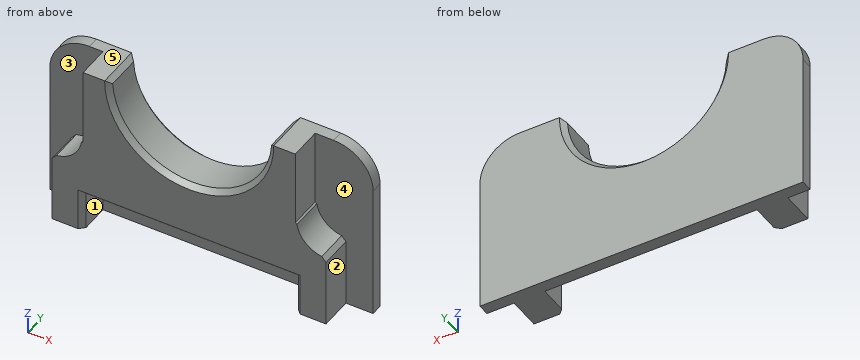
```python
from build123d import *

# Parameters (mm, degrees)
F0_W         = 124.8875334859
F0_H         = 67.7581354976
F1_DEPTH     = 4.445
F2_R         = 15.24
F4_DEPTH     = 12.7
F6_DEPTH     = 50.8
F8_DEPTH     = 12.7
F9_T1_DEPTH  = 26.6729642247
F9_T3_DEPTH  = 19.5947973283
F9_T5_DEPTH  = 81.9930359721
F9_T7_DEPTH  = 17.2644261819
F9_T10_ANGLE = 198.2651986278
F9_T12_ANGLE = 198.2651986278
F9_T16_DEPTH = 17.2644261819
F9_T21_DEPTH = 17.2644261819
F9_T27_DEPTH = 86.8920920642
F9_T31_DEPTH = 19.5947973283
F9_T38_DEPTH = 19.5947973283
F9_T42_DEPTH = 86.8920920642


# Not quite as in the source:
# - a fillet or chamfer that OpenCascade refuses, or shapes differently, is made with other operations: its cross-section is extruded or revolved along the edge and cut away or added


with BuildPart() as f1:
    # F0 (on Front) → F1 (new body)
    with BuildSketch(Plane.XZ):
        with Locations((0.9489916265, 33.8790677488)):
            Rectangle(F0_W, F0_H)
    extrude(amount=F1_DEPTH)

    # F2
    f2_edges = [f1.edges().sort_by_distance(p)[0] for p in [
        (-61.494775, -2.2225, 67.758135),
        (63.392758, -2.2225, 67.758135),
    ]]
    fillet(f2_edges, radius=F2_R)

    # F3 (on face) → F4 (join)
    with BuildSketch(Plane.XZ.offset(4.445)):
        Polygon((40.9965217113, 67.7581354976), (-40.9965142608, 67.7581354976), (-40.9965142608, 39.0565320849), (-40.9965142608, 14.6957412362), (40.9965217113, 14.6957412362), (40.9965217113, 39.4814237952), align=None)
        Polygon((-40.9965142608, 14.6957412362), (-40.9965142608, 39.0565320849), (-52.9372058809, 39.0565320849), (-52.9372058809, 0), (-40.9965142608, 0), align=None)
        Polygon((52.8750233352, 39.4814237952), (40.9965217113, 39.4814237952), (40.9965217113, 14.6957412362), (40.9965217113, 0), (52.8750233352, 0), align=None)
    extrude(amount=F4_DEPTH)

    # F5 (on face) → F6 (cut)
    with BuildSketch(Plane.XZ.offset(17.145)):
        with BuildLine():
            ThreePointArc((-30.7849538809, 67.7581354976), (0, 36.9731816167), (30.7849538809, 67.7581354976))
            Line((30.7849538809, 67.7581354976), (-30.7849538809, 67.7581354976))
        make_face()
        with BuildLine():
            Line((-30.7849538809, 67.7581354976), (30.7849538809, 67.7581354976))
            ThreePointArc((30.7849538809, 67.7581354976), (0, 98.5430893784), (-30.7849538809, 67.7581354976))
        make_face()
    extrude(amount=-F6_DEPTH, mode=Mode.SUBTRACT)

    # F7 (on face) → F8 (cut)
    with BuildSketch(Plane.XZ.offset(17.145)):
        with BuildLine():
            ThreePointArc((-52.9372058809, 27.6993892785), (-44.9064931875, 31.0258193916), (-41.5800630744, 39.0565320849))
            Line((-41.5800630744, 39.0565320849), (-52.9372058809, 39.0565320849))
            Line((-52.9372058809, 39.0565320849), (-52.9372058809, 27.6993892785))
        make_face()
        with BuildLine():
            Line((52.8750233352, 39.4814237952), (41.5178805288, 39.4814237952))
            ThreePointArc((41.5178805288, 39.4814237952), (44.8443106419, 31.4507111019), (52.8750233352, 28.1242809888))
            Line((52.8750233352, 28.1242809888), (52.8750233352, 39.4814237952))
        make_face()
    extrude(amount=-F8_DEPTH, mode=Mode.SUBTRACT)

    # F9: chamfer of 1.905 on 11 edges, made by hand

    # F9_s2 → F9_t1 (cut)
    with BuildSketch(Plane.XZ.offset(-4.7639821123)):
        with BuildLine():
            Line((-32.6343999444, 67.7581354976), (-30.7326373381, 65.964148961))
            ThreePointArc((-30.7326373381, 65.964148961), (-30.7710738122, 66.8337968736), (-30.7849538809, 67.7581354976))
            Line((-30.7849538809, 67.7581354976), (-32.6343999444, 67.7581354976))
        make_face()
        with BuildLine():
            Line((30.7326373381, 65.964148961), (32.6343999444, 67.7581354976))
            Line((32.6343999444, 67.7581354976), (30.7849538809, 67.7581354976))
            ThreePointArc((30.7849538809, 67.7581354976), (30.7710738122, 66.8337968736), (30.7326373381, 65.964148961))
        make_face()
    extrude(amount=F9_T1_DEPTH, mode=Mode.SUBTRACT)

    # F9_s4 → F9_t3 (cut)
    with BuildSketch(Plane.XY.offset(-4.8990560921)):
        Polygon((-42.9015142608, -17.145), (-40.9965142608, -15.24), (-40.9965142608, -17.145), align=None)
        Polygon((42.9015217113, -17.145), (40.9965217113, -15.24), (40.9965217113, -17.145), align=None)
    extrude(amount=F9_T3_DEPTH, mode=Mode.SUBTRACT)

    # F9_s6 → F9_t5 (cut)
    with BuildSketch(Plane.YZ.offset(-40.9965142608)):
        Polygon((-17.145, 16.6007412362), (-15.24, 14.6957412362), (-17.145, 14.6957412362), align=None)
    extrude(amount=F9_T5_DEPTH, mode=Mode.SUBTRACT)

    # F9_s8 → F9_t7 (cut)
    with BuildSketch(Plane.XZ.offset(4.445)):
        with BuildLine():
            Line((52.8750233352, 26.356813065), (51.2436612422, 28.24205769))
            ThreePointArc((51.2436612422, 28.24205769), (52.0302167258, 28.1557452496), (52.8750233352, 28.1242809888))
            Line((52.8750233352, 28.1242809888), (52.8750233352, 26.356813065))
        make_face()
        with BuildLine():
            Line((-52.9372058809, 25.9319213547), (-51.3058437879, 27.8171659797))
            ThreePointArc((-51.3058437879, 27.8171659797), (-52.0923992715, 27.7308535393), (-52.9372058809, 27.6993892785))
            Line((-52.9372058809, 27.6993892785), (-52.9372058809, 25.9319213547))
        make_face()
    extrude(amount=F9_T7_DEPTH, mode=Mode.SUBTRACT)

    # F9_s9 → F9_t10 (revolve, cut)
    with BuildSketch(Plane(origin=(10.6182323587, 0, 66.0511732612), x_dir=(0, 1, 0), z_dir=(0.1587198459, 0, 0.9873236605))):
        Polygon((-15.24, 41.539514704), (-17.145, 43.444514704), (-17.145, 41.539514704), align=None)
    revolve(axis=Axis((0, -17.145, 67.7581354976), (0, -1, 0)), revolution_arc=F9_T10_ANGLE, mode=Mode.SUBTRACT)

    # F9_s11 → F9_t12 (revolve, cut)
    with BuildSketch(Plane(origin=(10.6182323587, 0, 66.0511732612), x_dir=(0, 1, 0), z_dir=(0.1587198459, 0, 0.9873236605))):
        Polygon((0, 43.444514704), (-1.905, 41.539514704), (0, 41.539514704), align=None)
    revolve(axis=Axis((0, 0, 67.7581354976), (0, -1, 0)), revolution_arc=F9_T12_ANGLE, mode=Mode.SUBTRACT)


with BuildPart() as f9_tool14:
    # F9_s15 → F9_t16 (new body)
    with BuildSketch(Plane.XZ.offset(21.7094261819)):
        with BuildLine():
            Line((41.63565723, 37.8500617022), (39.750412605, 39.4814237952))
            Line((39.750412605, 39.4814237952), (41.5178805288, 39.4814237952))
            ThreePointArc((41.5178805288, 39.4814237952), (41.5493447896, 38.6366171858), (41.63565723, 37.8500617022))
        make_face()
    extrude(amount=-F9_T16_DEPTH)

    split(bisect_by=Plane.YZ.offset(40.9965217113), keep=Keep.TOP)


with BuildPart() as f1_1:
    add(f1.part)

    # F9_t13: cut F9_tool14
    add(f9_tool14.part, mode=Mode.SUBTRACT)


with BuildPart() as f9_tool19:
    # F9_s20 → F9_t21 (new body)
    with BuildSketch(Plane.XZ.offset(21.7094261819)):
        with BuildLine():
            Line((-39.8125951507, 39.0565320849), (-41.6978397756, 37.4251699919))
            ThreePointArc((-41.6978397756, 37.4251699919), (-41.6115273352, 38.2117254755), (-41.5800630744, 39.0565320849))
            Line((-41.5800630744, 39.0565320849), (-39.8125951507, 39.0565320849))
        make_face()
    extrude(amount=-F9_T21_DEPTH)

    split(bisect_by=Plane.YZ.offset(-40.9965142608), keep=Keep.BOTTOM)


with BuildPart() as f1_2:
    add(f1_1.part)

    # F9_t18: cut F9_tool19
    add(f9_tool19.part, mode=Mode.SUBTRACT)


with BuildPart() as f9_tool25:
    # F9_s26 → F9_t27 (new body)
    with BuildSketch(Plane.YZ.offset(-45.8955703528)):
        Polygon((-17.145, 16.6007412362), (-15.24, 14.6957412362), (-17.145, 14.6957412362), align=None)
    extrude(amount=F9_T27_DEPTH)

    split(bisect_by=Plane.YZ.offset(-40.9965142608), keep=Keep.BOTTOM)


with BuildPart() as f9_tool29:
    # F9_s30 → F9_t31 (new body)
    with BuildSketch(Plane.XY):
        Polygon((-42.9015142608, -17.145), (-40.9965142608, -15.24), (-40.9965142608, -17.145), align=None)
    extrude(amount=F9_T31_DEPTH)

    split(bisect_by=Plane.XY.offset(14.6957412362), keep=Keep.TOP)


with BuildPart() as f9_tool25_1:
    add(f9_tool25.part)

    # F9_t33: intersect F9_tool29
    add(f9_tool29.part, mode=Mode.INTERSECT)


with BuildPart() as f1_3:
    add(f1_2.part)

    # F9_t23: cut F9_tool25
    add(f9_tool25_1.part, mode=Mode.SUBTRACT)


with BuildPart() as f9_tool36:
    # F9_s37 → F9_t38 (new body)
    with BuildSketch(Plane.XY.offset(19.5947973283)):
        Polygon((42.9015217113, -17.145), (40.9965217113, -15.24), (40.9965217113, -17.145), align=None)
    extrude(amount=-F9_T38_DEPTH)

    split(bisect_by=Plane.XY.offset(14.6957412362), keep=Keep.TOP)


with BuildPart() as f9_tool40:
    # F9_s41 → F9_t42 (new body)
    with BuildSketch(Plane.YZ.offset(-40.9965142608)):
        Polygon((-17.145, 16.6007412362), (-15.24, 14.6957412362), (-17.145, 14.6957412362), align=None)
    extrude(amount=F9_T42_DEPTH)

    split(bisect_by=Plane.YZ.offset(40.9965217113), keep=Keep.TOP)


with BuildPart() as f9_tool36_1:
    add(f9_tool36.part)

    # F9_t44: intersect F9_tool40
    add(f9_tool40.part, mode=Mode.INTERSECT)


with BuildPart() as f1_4:
    add(f1_3.part)

    # F9_t34: cut F9_tool36
    add(f9_tool36_1.part, mode=Mode.SUBTRACT)


solid = f1_4.part
```
Build history of the part. All positions in model axes, mm. Face numbers are marked on the shaded views. A direction names the side the tool comes from. Round coordinates to 2 decimals unless told otherwise and drop trailing zeros. Write each loop counter-clockwise with the first axis right and the second up, starting at its lowest first coordinate (ties: lowest second). Pieces come first, ordered by that corner, then holes. Notation, with made-up numbers: (40, -24.75) - (57, -24.75) arc R21 ccw to (57, -5.75) - close; hole circle Ø2 at (-24, 15.25). An arc over 180 degrees is marked (long way). Write each question's results on one line, items separated by ' | '. Start each with the question number.
Item 1: Drop flat-ended pins along their axis: P1, Ø6, axis at x = -56, z = 47.5, coming from the -Y side (3 decimals); P2, Ø5.5, axis at x = 6.5, y = -10, coming from the -Z side; P3, Ø24.5, axis at x = 53.5, z = 31, coming from the -Y side (3 decimals); P4, Ø1.5, axis at y = -9, z = 30, coming from the +X side. Give the stop position or say it passes through.
Item 2: Saw through at C-C (y = -12.25). Write the cut outline in (x, z), and give its area (3 significant figures).
Item 3: Wall check: L1, parallel to X at y = -15, z = 3.5; L2, parallel to Y at x = -49, z = 51 (3 decimals); L3, parallel to X at y = -15.25, z = 21.5. Give the ranges that are in metal, low to high. Write a range as [from, to].
Item 4: Saw through at B-B (z = 20.5). Write the cut outline in (x, y) (3 decimals).
Item 5: Mould opens along X. For the marked faces 1, 2 and 3 say: pulls with the +X half, pulls with the -X half, needs draft (parallel to the pull), parting line crosses it, or undercut.
Item 6: Saw through at D-D (z = 13). Write the cut outline in (x, y) (3 decimals).
Item 7: Saw through at A-A (x = 0). Write the cut outline in (y, z) (3 decimals).
Item 8: Which spindle directions (+Z, -Z, +X, -X, +Y, -Y) get a long thin tool onto all of the face, cutting with end or side? Do the marked faces 4 and 5. Say none if no direction does.
Results are:
1) P1: stops at y = -4.445 | P2: stops at z = 14.7 | P3: stops at y = -17.145 | P4: stops at x = 47.95
2) outline: (-52.94, 0) - (-41, 0) - (-41, 14.7) - (41, 14.7) - (41, 0) - (52.88, 0) - (52.88, 26.36) - (51.24, 28.24) arc R11.36 cw to (41.64, 37.85) - (41, 38.4) - (41, 67.76) - (32.63, 67.76) - (30.73, 65.96) arc R30.78 cw to (-30.73, 65.96) - (-32.63, 67.76) - (-41, 67.76) - (-41, 38.03) - (-41.7, 37.43) arc R11.36 cw to (-51.31, 27.82) - (-52.94, 25.93) - close | area: 3,590 mm²
3) L1: x = [-52.94, -41], [41, 52.88] | L2: y = [-4.445, 0] | L3: x = [-52.94, 52.88]
4) outline: (-61.495, -4.445) - (-52.937, -4.445) - (-52.937, -17.145) - (52.875, -17.145) - (52.875, -4.445) - (63.393, -4.445) - (63.393, 0) - (-61.495, 0) - close
5) face 1: undercut | face 2: pulls with the +X half | face 3: needs draft
6) outline: (-61.495, -4.445) - (-52.937, -4.445) - (-52.937, -17.145) - (-42.902, -17.145) - (-40.997, -15.24) - (-40.997, -4.445) - (40.997, -4.445) - (40.997, -15.24) - (42.902, -17.145) - (52.875, -17.145) - (52.875, -4.445) - (63.393, -4.445) - (63.393, 0) - (-61.495, 0) - close
7) outline: (-17.145, 16.601) - (-15.24, 14.696) - (-4.445, 14.696) - (-4.445, 0) - (0, 0) - (0, 35.068) - (-1.905, 36.973) - (-15.24, 36.973) - (-17.145, 35.068) - close
8) face 4: +Z, +X, -Y | face 5: +Z, +X, -X, +Y, -Y
